Read the model definition and answer for the solid it produces. Units are mm, in the model's axes. A direction names the side the tool comes from. Round coordinates to 2 decimals unless told otherwise and drop trailing zeros. Loops run counter-clockwise (first coordinate to the right, second up) from the corner with the lowest first, then second, coordinate; pieces in that order, holes last. Notation, with made-up numbers: (15.5, 60.25) - (35.5, 60.25) arc R32 cw to (35.5, 89.25) - close; hole circle Ø9 at (-20, 10.25). An arc over 180 degrees is marked (long way). Use one line per item in the form item = value. Start each with the question number.
```python
from build123d import *

# Parameters (mm, degrees)
BOSS_EXTRUDE1_DEPTH     = 41
SKETCH3_W               = 25.226628976
SKETCH3_H               = 35
CUT_EXTRUDE2_DEPTH      = 39
CUT_EXTRUDE2_DEPTH_BACK = 1
CUT_EXTRUDE3_DEPTH      = 39
SKETCH5_R               = 2.5
CUT_EXTRUDE4_DEPTH      = 42
SKETCH6_R               = 2.5
CUT_EXTRUDE5_DEPTH      = 42.0000001
FILLET1_R               = 2


with BuildPart() as part:
    # Sketch1 → Boss-Extrude1 (new body)
    with BuildSketch(Plane.XY):
        with BuildLine():
            Line((-21.875, 0), (-41.755779843, 2.180502889))
            ThreePointArc((-41.755779843, 2.180502889), (-46.717396797, 6.03211956), (-45.524663567, 12.198964882))
            Line((-45.524663567, 12.198964882), (-21.875, 38))
            Line((-21.875, 38), (21.875, 38))
            Line((21.875, 38), (45.524663567, 12.198964882))
            ThreePointArc((45.524663567, 12.198964882), (46.717396797, 6.03211956), (41.755779843, 2.180502889))
            Line((41.755779843, 2.180502889), (21.875, 0))
            Line((21.875, 0), (-21.875, 0))
        make_face()
    extrude(amount=BOSS_EXTRUDE1_DEPTH)

    # Sketch3 → Cut-Extrude2 (cut, two sides)
    with BuildSketch(Plane(origin=(0, 0, 0), x_dir=(1, 0, 0), z_dir=(0, 1, 0))) as cut_extrude2_sk:
        with Locations((34.488314488, -20.5)):
            Rectangle(SKETCH3_W, SKETCH3_H)
        with Locations((-34.488314488, -20.5)):
            Rectangle(SKETCH3_W, SKETCH3_H)
    extrude(amount=CUT_EXTRUDE2_DEPTH, mode=Mode.SUBTRACT)
    extrude(cut_extrude2_sk.sketch, amount=-CUT_EXTRUDE2_DEPTH_BACK, mode=Mode.SUBTRACT)

    # Sketch4 → Cut-Extrude3 (cut, through all)
    with BuildSketch(Plane.XZ):
        with BuildLine():
            Line((-17.5, 20), (-17.5, 41))
            Line((-17.5, 41), (17.5, 41))
            Line((17.5, 41), (17.5, 20))
            ThreePointArc((17.5, 20), (0, 2.5), (-17.5, 20))
        make_face()
    extrude(amount=-CUT_EXTRUDE3_DEPTH, mode=Mode.SUBTRACT)

    # Sketch5 → Cut-Extrude4 (cut, through all)
    with BuildSketch(Plane(origin=(0, 0, 0), x_dir=(-1, 0, 0), z_dir=(0, 0, -1))):
        with Locations((0, 28)):
            Circle(SKETCH5_R)
        with Locations((0, 10)):
            Circle(SKETCH5_R)
    extrude(amount=-CUT_EXTRUDE4_DEPTH, mode=Mode.SUBTRACT)

    # Sketch6 → Cut-Extrude5 (cut, through all)
    with BuildSketch(Plane.XY.offset(41)):
        with Locations((-41.101628976, 8.144736842)):
            Circle(SKETCH6_R)
    cut_extrude5 = extrude(amount=-CUT_EXTRUDE5_DEPTH, mode=Mode.SUBTRACT)

    # Mirror1: Cut-Extrude5 across plane
    add(cut_extrude5.mirror(Plane(origin=(0, 0, 0), x_dir=(0, 0, 1), z_dir=(1, 0, 0))), mode=Mode.SUBTRACT)

    # Fillet1
    fillet1_edges = [part.edges().sort_by_distance(p)[0] for p in [
        (21.875, 19, 3),
        (21.875, 19, 38),
        (-21.875, 19, 38),
        (-21.875, 19, 3),
    ]]
    fillet(fillet1_edges, radius=FILLET1_R)


solid = part.part
```
1) A cutting plane is placed at D-D on y = 32.5. Write down the section's boundary in (x, z) (3 decimals), plus the area to 3 significant figures.
2) A cutting plane is placed at C-C on x = -31. Write down the section's boundary in (y, z), plus the area to 3 significant figures.
3) Determine the mould class of faces 1 (the flat face through (-33, 14, 3)), 2 (the flat face through (1, 19, 0)), 3 (the flat face through (0, 38, 2)) for opening direction Z: +Z half, -Z half, draft (parallel to the pull), parting line (faces both ways), or undercut.
4) Flat-ended cylindrical pins translate along their axes: pin 1 (17 mm diameter, centred on y = 21, z = 25.5, fed in from +X) (3 decimals); pin 2 (15.5 mm diameter, centred on y = 11.5, z = 27.5, fed in from -X) (3 decimals); pin 3 (8 mm diameter, centred on x = 0, y = 10, fed in from +Z). Find the tip coordinate at first contact, or state that the pin passes through.
5) A cutting plane is placed at A-A on x = 0. Write down the section's boundary in (y, z), plus the area to 3 significant figures.
6) A cutting plane is placed at B-B on z = 24.5. Write down the section's boundary in (x, y) (3 decimals).
7) Straight lines are drawn through the part: line 1 (X direction, y = 14.5, z = 25.5) (3 decimals); line 2 (Z direction, x = 36.5, y = 2.5); line 3 (Y direction, x = 0, z = 1). For each, find the intervals that lie inside material, in ascending order. Write a range as from..to.
8) For faces 4 (the flat face through (17.5, 19, 31)), 5 (the cylindrical face through (22.445, 19.266, 3.601)), 6 (the cylindrical face through (46.75, 6.12, 39.48)), determine the directions among +Z, -Z, +X, -X, +Y, -Y from which every point of the face is accessible in a straight line to the end or side of a thin tool.
Checks:
q1.outline = (-26.916, 0) - (26.916, 0) - (26.916, 3) - (23.875, 3) arc R2 cw to (21.875, 5) - (21.875, 36) arc R2 cw to (23.875, 38) - (26.916, 38) - (26.916, 41) - (17.5, 41) - (17.5, 20) arc R17.5 cw to (-17.5, 20) - (-17.5, 41) - (-26.916, 41) - (-26.916, 38) - (-23.875, 38) arc R2 cw to (-21.875, 36) - (-21.875, 5) arc R2 cw to (-23.875, 3) - (-26.916, 3) - close
q1.area = 642 mm²
q2.outline = (1, 0) - (28.04, 0) - (28.04, 3) - (1, 3) - close; (1, 38) - (28.04, 38) - (28.04, 41) - (1, 41) - close
q2.area = 162 mm²
q3.face_1 = undercut
q3.face_2 = -Z half
q3.face_3 = draft
q4.pin_1 = 21.875
q4.pin_2 = -21.875
q4.pin_3 = 2.96
q5.outline = (0, 0) - (7.5, 0) - (7.5, 2.5) - (0, 2.5) - close; (12.5, 0) - (25.5, 0) - (25.5, 2.5) - (12.5, 2.5) - close; (30.5, 0) - (38, 0) - (38, 2.5) - (30.5, 2.5) - close
q5.area = 70.0 mm²
q6.outline = (-21.875, 0) - (-17.5, 0) - (-17.5, 38) - (-21.875, 38) - close; (17.5, 0) - (21.875, 0) - (21.875, 38) - (17.5, 38) - close
q7.line_1 = -21.875..-17.5, 17.5..21.875
q7.line_2 = 0..3, 38..41
q7.line_3 = 0..7.5, 12.5..25.5, 30.5..38
q8.face_4 = +Z, +Y, -Y
q8.face_5 = +X, +Y, -Y
q8.face_6 = +Z, -Z, +X
